```python
from build123d import *

# Parameters (mm, degrees)
SKETCH009_W     = 68
SKETCH009_H     = 80
PAD005_DEPTH    = 3
SKETCH010_R     = 23
POCKET004_DEPTH = 3
SKETCH011_W     = 68
SKETCH011_H     = 5
PAD006_DEPTH    = 30
SKETCH024_R     = 1
POCKET017_DEPTH = 5
SKETCH025_R     = 1
POCKET018_DEPTH = 5
SKETCH026_R     = 0.5
POCKET019_DEPTH = 10
CHAMFER002_SIZE = 0.8


with BuildPart() as part:
    # Sketch009 → Pad005 (new body)
    with BuildSketch(Plane.XY):
        with Locations((34, 40)):
            Rectangle(SKETCH009_W, SKETCH009_H)
    extrude(amount=PAD005_DEPTH)

    # Sketch010 (on Face6 of Pad005) → Pocket004 (cut)
    with BuildSketch(Plane.XY.offset(3)):
        with Locations((34, 40)):
            Circle(SKETCH010_R)
    extrude(amount=-POCKET004_DEPTH, mode=Mode.SUBTRACT)

    # Sketch011 (on Face4 of Pocket004) → Pad006 (join)
    with BuildSketch(Plane(origin=(0, 0, 0), x_dir=(1, 0, 0), z_dir=(0, 0, -1))):
        with Locations((34, -2.5)):
            Rectangle(SKETCH011_W, SKETCH011_H)
        with Locations((34, -77.5)):
            Rectangle(SKETCH011_W, SKETCH011_H)
    extrude(amount=PAD006_DEPTH)

    # Sketch024 (on Face4 of Pad006) → Pocket017 (cut)
    with BuildSketch(Plane.XZ):
        with Locations((33, -27)):
            Circle(SKETCH024_R)
    extrude(amount=-POCKET017_DEPTH, mode=Mode.SUBTRACT)

    # Sketch025 (on Face15 of Pocket017) → Pocket018 (cut)
    with BuildSketch(Plane(origin=(0, 80, 0), x_dir=(-1, 0, 0), z_dir=(0, 1, 0))):
        with Locations((-33, -27)):
            Circle(SKETCH025_R)
    extrude(amount=-POCKET018_DEPTH, mode=Mode.SUBTRACT)

    # Sketch026 (on Face5 of Pocket018) → Pocket019 (cut)
    with BuildSketch(Plane.XY.offset(3)):
        with Locations((22.6, 2.5)):
            Circle(SKETCH026_R)
        with Locations((45.3, 2.5)):
            Circle(SKETCH026_R)
        with Locations((22.6, 77.5)):
            Circle(SKETCH026_R)
        with Locations((45.3, 77.5)):
            Circle(SKETCH026_R)
    extrude(amount=-POCKET019_DEPTH, mode=Mode.SUBTRACT)

    # Chamfer002
    chamfer002_edges = [part.edges().sort_by_distance(p)[0] for p in [
        (22.1, 2.5, 3),
        (44.8, 2.5, 3),
        (44.8, 77.5, 3),
        (22.1, 77.5, 3),
    ]]
    chamfer(chamfer002_edges, length=CHAMFER002_SIZE)


with BuildPart() as part_1:
    # Body004 placement: moved
    add(part.part.moved(Location((7, 10, -5))))


with BuildPart() as part_2:
    # Clone001 placement: moved
    add(part_1.part.moved(Location((3, 0, 0))))


with BuildPart() as part_3:
    # Body005 placement: moved
    add(part_2.part.moved(Location((217, 0, 0))))


solid = part_3.part
```
The model under review builds one solid part; all positions refer to its coordinate system, in mm. A direction names the side the tool comes from. Coordinates: 2 decimals unless noted, no trailing zeros. Write each loop counter-clockwise with the first axis right and the second up, starting at its lowest first coordinate (ties: lowest second). Pieces come first, ordered by that corner, then holes. Notation, with made-up numbers: (68, 87) - (101, 87) arc R14 ccw to (101, 113) - close; hole circle Ø1 at (81.25, -23). An arc over 180 degrees is marked (long way). Answer in a Markdown table with one row per item. Add a question column.
Q1. Draft analysis for pull direction X (two halves, no side actions). For faces 3 (the face through (261, 12, -35)), 4 (the face through (261, 88, -32)), 5 (the face through (227, 50, -4)), 6 (the face through (295, 50, -4)), state which applies: +X half, -X half, draft (parallel to the pull), parting line (faces both ways), or undercut.
Q2. Consider section B-B on y = 50. Give the boundary of the cut face in (x, z).
Q3. Consider section C-C on z = -28. Give the boundary of the cut face in (x, y), then the cut area to 3 significant figures.
Q4. To check wall thickness, follow line 1 along Y through (x, z) = (249.6, -9.75); line 2 along Y through (x, z) = (275.5, -9); line 3 along Y through (x, z) = (261, -2.95). State the ranges of each line that lie inside material, in increasing order. Write a range as from..to.
Q5. Consider section A-A on z = -32. Give the boundary of the cut face in (x, y), then the cut area to 3 significant figures.
Q6. Clearance check with flat-ended pins moving along their axes: pin 1 (8 mm diameter, centred on x = 276, y = 67, fed in from -Z); pin 2 (3 mm diameter, centred on x = 260, z = -32, fed in from -Y); pin 3 (1.1 mm diameter, centred on x = 272.5, y = 87.5, fed in from +Z); pin 4 (0.5 mm diameter, centred on x = 272.5, y = 12.5, fed in from +Z). State where each tip first meets the part, or that it passes through.
Q7. Consider section D-D on x = 260. Give the boundary of the cut face in (y, z), then the cut area to 3 significant figures.
Q8. For faces 1 (the face through (261, 74, -5)), 2 (the face through (261, 87, -35)), list the 3-axis set-ups (+Z, -Z, +X, -X, +Y, -Y) from which the entire face can be reached by the end or side of a thin tool; tool diameter is ignored.
Answers below:
| question | item | result |
|---|---|---|
| 1 | face 3 | draft |
| 1 | face 4 | undercut |
| 1 | face 5 | -X half |
| 1 | face 6 | +X half |
| 2 | outline | (227, -5) - (238, -5) - (238, -2) - (227, -2) - close; (284, -5) - (295, -5) - (295, -2) - (284, -2) - close |
| 3 | outline | (227, 10) - (295, 10) - (295, 15) - (227, 15) - close; (227, 85) - (295, 85) - (295, 90) - (227, 90) - close |
| 3 | area | 680 mm² |
| 4 | line 1 | 10..12, 13..15, 85..87, 88..90 |
| 4 | line 2 | 10..15, 85..90 |
| 4 | line 3 | 10..27, 73..90 |
| 5 | outline | (227, 10) - (259, 10) - (259, 15) - (227, 15) - close; (227, 85) - (259, 85) - (259, 90) - (227, 90) - close; (261, 10) - (295, 10) - (295, 15) - (261, 15) - close; (261, 85) - (295, 85) - (295, 90) - (261, 90) - close |
| 5 | area | 660 mm² |
| 6 | pin 1 | z = -5 |
| 6 | pin 2 | y = 10 |
| 6 | pin 3 | z = -2.55 |
| 6 | pin 4 | z = -12 |
| 7 | outline | (10, -35) - (15, -35) - (15, -33) - (10, -33) - close; (10, -31) - (15, -31) - (15, -5) - (27.02, -5) - (27.02, -2) - (10, -2) - close; (72.98, -5) - (85, -5) - (85, -31) - (90, -31) - (90, -2) - (72.98, -2) - close; (85, -35) - (90, -35) - (90, -33) - (85, -33) - close |
| 7 | area | 382 mm² |
| 8 | face 1 | -Z, +X, -X |
| 8 | face 2 | -Z, +X, -X, +Y, -Y |
